Autodesk Inventor part; units mm, degrees
ref_plane "YZ Plane" through (0, 0, 0) normal (1, 0, 0) x (0, 1, 0)
ref_plane "XZ Plane" through (0, 0, 0) normal (0, 1, 0) x (-1, 0, 0)
ref_plane "XY Plane" through (0, 0, 0) normal (0, 0, 1) x (1, 0, 0)
sketch "Sketch1" plane through (0, 0, 0) normal (0, 0, 1) x (1, 0, 0)
  line L0 (-11, -29.75) -> (11, -29.75) construction
  line L1 (14.5, -26.25) -> (14.5, 26.25) construction
  line L2 (11, 29.75) -> (-11, 29.75) construction
  line L3 (-14.5, 26.25) -> (-14.5, -26.25) construction
  line L4 (-14.5, -29.75) -> (14.5, 29.75) construction
  line L5 (14.5, -29.75) -> (-14.5, 29.75) construction
  arc A0 (-11, 29.75) -> (-14.5, 26.25) centre (-11, 26.25) ccw construction
  arc A1 (14.5, 26.25) -> (11, 29.75) centre (11, 26.25) ccw construction
  arc A2 (11, -29.75) -> (14.5, -26.25) centre (11, -26.25) ccw
  arc A3 (-14.5, -26.25) -> (-11, -29.75) centre (-11, -26.25) ccw construction
  line L6 (-17.6, -35) -> (17.6, -35)
  line L7 (20.1, -32.5) -> (20.1, 34.5)
  line L8 (17.6, 37) -> (-17.6, 37)
  line L9 (-20.1, 34.5) -> (-20.1, -32.5)
  line L10 (-20.1, -35) -> (20.1, 37) construction
  line L11 (20.1, -35) -> (-20.1, 37) construction
  line L12 (-20.1, 34.5) -> (-17.6, 37)
  line L13 (-20.1, -32.5) -> (-17.6, -35)
  line L14 (17.6, -35) -> (20.1, -32.5)
  line L15 (17.6, 37) -> (20.1, 34.5)
  circle A4 centre (0, -15.25) radius 14 construction
  circle A5 centre (-17.3, -19.25) radius 1.3
  circle A6 centre (-17.3, 2.75) radius 1.3
  circle A7 centre (-17.3, 24.75) radius 1.3
  circle A8 centre (-11, 32.55) radius 1.3
  line L16 (0, -15.25) -> (0, -1.25) construction
  circle A9 centre (17.3, -19.25) radius 1.3
  circle A10 centre (17.3, 2.75) radius 1.3
  circle A11 centre (17.3, 24.75) radius 1.3
  circle A12 centre (11, 32.55) radius 1.3
  line L17 (-11, 30) -> (11, 30)
  arc A13 (14.75, 26.25) -> (11, 30) centre (11, 26.25) ccw
  line L18 (14.75, 26.25) -> (14.75, -26.25)
  arc A14 (11, -30) -> (14.75, -26.25) centre (11, -26.25) ccw
  line L19 (11, -30) -> (-11, -30)
  arc A15 (-14.75, -26.25) -> (-11, -30) centre (-11, -26.25) ccw
  line L20 (-14.75, -26.25) -> (-14.75, 26.25)
  arc A16 (-11, 30) -> (-14.75, 26.25) centre (-11, 26.25) ccw
  point P0 (0, 0)
  point P1 (0, 1)
  point P2 (0, 29.75)
  dimension "d14" = 28
  dimension "d0" = 29
  dimension "d1" = 59.5
  dimension "d2" = 3.5
  dimension "d3" = 40.2
  dimension "d4" = 72
  dimension "d6" = 2.5
  dimension "d7" = 2.5
  dimension "d8" = 2.5
  dimension "d9" = 2.5
  dimension "d10" = 2.5
  dimension "d11" = 2.5
  dimension "d12" = 2.5
  dimension "d13" = 2.5
  dimension "d15" = 45
  dimension "d16" = 2.6
  dimension "d17" = 17.3
  dimension "d18" = 4
  dimension "d19" = 2.6
  dimension "d20" = 22
  dimension "d21" = 2.6
  dimension "d22" = 22
  dimension "d24" = 2.6
  dimension "d26" = 7.8
  dimension "d27" = 11
  dimension "d28" = 1
  dimension "d51" = 0.25
extrude "Extrusion1" add sketch "Sketch1" along normal blind 6
sketch "Sketch2" plane through (0, 0, 6) normal (0, 0, 1) x (1, 0, 0)
  line L0 (26.1, 28) -> (26.1, 20)
  line L1 (20.1, -32.5) -> (20.1, 34.5)
  line L2 (26.1, 20) -> (20.1, 20)
  line L3 (26.1, 28) -> (20.1, 28)
  line L4 (-14.5, 0) -> (14.5, 0) construction
  line L5 (0, 29.4068) -> (0, -29.4068) construction
  line L6 (-26.1, 28) -> (-26.1, 20)
  line L7 (-26.1, 20) -> (-20.1, 20)
  line L8 (-26.1, 28) -> (-20.1, 28)
  line L9 (26.1, -28) -> (26.1, -20)
  line L10 (26.1, -20) -> (20.1, -20)
  line L11 (26.1, -28) -> (20.1, -28)
  line L12 (-26.1, -20) -> (-20.1, -20)
  line L13 (-26.1, -28) -> (-26.1, -20)
  line L14 (-26.1, -28) -> (-20.1, -28)
  line L15 (-20.1, 28) -> (-20.1, 20)
  line L16 (-20.1, 34.5) -> (-20.1, -32.5)
  line L17 (-20.1, -20) -> (-20.1, -28)
  line L18 (-20.1, 34.5) -> (-20.1, -32.5)
  point P0 (0, 0)
  point P1 (26.1, 24)
  point P2 (20.1, -20)
  point P3 (20.1, -28)
  point P4 (0, 0)
  dimension "d31" = 24
  dimension "d32" = 8
  dimension "d33" = 6
extrude "Extrusion2" add sketch "Sketch2" against normal up to surface (6 mm away)
fillet "Fillet1" radius 5 8 edges at (20.1, 28, 3) (-20.1, 28, 3) (-20.1, -20, 3) (-20.1, -28, 3) (20.1, -28, 3) (20.1, 20, 3) (20.1, -20, 3) (-20.1, 20, 3)
sketch "Sketch3" plane through (-26.1, 20, 6) normal (-1, 0, 0) x (0, 0, 1)
  line L0 (-6, 0) -> (-6, 8) construction
  line L1 (0, 0) -> (-6, 0) construction
  line L2 (0, 8) -> (0, 0) construction
  line L3 (0, 8) -> (-6, 8) construction
  line L4 (0, 8) -> (-6, 0) construction
  circle A0 centre (-3, 4) radius 2
  line L5 (-6, -48) -> (-6, -40) construction
  line L6 (0, -48) -> (-6, -48) construction
  line L7 (0, -40) -> (0, -48) construction
  line L8 (0, -40) -> (-6, -40) construction
  line L9 (0, -40) -> (-6, -48) construction
  circle A1 centre (-3, -44) radius 2
  point P0 (-6, -20)
  dimension "d37" = 4
  dimension "d38" = 4
extrude "Extrusion3" cut sketch "Sketch3" against normal blind 6
mirror "Mirror1" about plane through (0, 0, 0) normal (1, 0, 0) of "Extrusion3"
thread "Thread1"
thread "Thread2"
thread "Thread3"
thread "Thread4"
equation "\"d7\" = d6"
equation "\"d8\" = d6"
equation "\"d9\" = d8"
equation "\"d10\" = d6"
equation "\"d11\" = d10"
equation "\"d12\" = d6"
equation "\"d13\" = d12"
properties part number "DynamixelServoMount" material "Aluminum 6061"
Can you work these out from the model? Positions are in its coordinate system, mm. A direction names the side the tool comes from. Coordinates: 2 decimals unless noted, no trailing zeros. Write each loop counter-clockwise with the first axis right and the second up, starting at its lowest first coordinate (ties: lowest second). Pieces come first, ordered by that corner, then holes.
Q1. Which directions (+Z, -Z, +X, -X, +Y, -Y) give clear straight access to the entire face, cutting with the end or side of a thin tool? Please do faces 1 (the face through (14.75, 0, 3)), 2 (the face through (20.1, 24, 3)), 3 (the face through (0, -35, 3)), 4 (the face through (-21.53, 18.5, 3.04)), 5 (the face through (-20.1, 34, 3)).
Results found:
face 1: +Z, -Z
face 2: +X
face 3: +Z, -Z, +X, -X, -Y
face 4: +Z, -Z, -X
face 5: +Z, -Z, -X, +Y
Q2. Imagine slicing it at B-B, the plane x = 21. List the corners of the cut face in (y, z) for me.
Results found:
outline: (-30.1, 0) - (-17.86, 0) - (-17.86, 6) - (-30.1, 6) - close; (17.86, 0) - (30.14, 0) - (30.14, 6) - (17.86, 6) - close; hole circle Ø4 at (-24, 3); hole circle Ø4 at (24, 3)
Q3. If we mould it in two halves opening along X, with no side actions, what happens to faces 6 (the face through (-16.7, -18.097, 2.958)), 7 (the face through (-26.1, 23, 5)), 8 (the face through (-16, 1, 0))? For each: +X half, -X half, draft (parallel to the pull), parting line (faces both ways), or undercut.
Results found:
face 6: undercut
face 7: -X half
face 8: draft
Q4. Imagine slicing it at C-C, the plane x = 8. List the corners of the cut face in (y, z) for me.
Results found:
outline: (-35, 0) - (-30, 0) - (-30, 6) - (-35, 6) - close; (30, 0) - (37, 0) - (37, 6) - (30, 6) - close
Q5. Please list where these lines run through material, in increasing order: L1, parallel to Y at x = 17.3, z = 1.95; L2, parallel to Y at x = 3, z = 3.4; L3, parallel to X at y = -21, z = 4.15.
Results found:
L1: y = -35 to -20.55, -17.95 to 1.45, 4.05 to 23.45, 26.05 to 37
L2: y = -35 to -30, 30 to 37
L3: x = -26.1 to -14.75, 14.75 to 26.1
Q6. For P1, Ø2, axis at y = 24, z = 3.5, coming from the -X side; P2, Ø0.8, axis at x = 25.5, z = 3, coming from the +Y side; P3, Ø1.5, axis at y = 12, z = 5, coming from the +X side, each with a flat end and sliding along its axis, tell me the tip position at first contact or that it passes through.
Results found:
P1: stops at x = -20.1
P2: stops at y = 28
P3: stops at x = 20.1
Q7. Imagine slicing it at A-A, the plane y = -24. List the corners of the cut face in (x, z) for me, plus the area to 3 significant figures.
Results found:
outline: (-26.1, 0) - (-14.75, 0) - (-14.75, 6) - (-26.1, 6) - (-26.1, 5) - (-20.1, 5) - (-20.1, 1) - (-26.1, 1) - close; (14.75, 0) - (26.1, 0) - (26.1, 1) - (20.1, 1) - (20.1, 5) - (26.1, 5) - (26.1, 6) - (14.75, 6) - close
area: 88.2 mm2
Q8. Imagine slicing it at D-D, the plane y = 24.75. List the corners of the cut face in (x, z) for me.
Results found:
outline: (-26.1, 0) - (-18.6, 0) - (-18.6, 6) - (-26.1, 6) - (-26.1, 4.85) - (-20.1, 4.85) - (-20.1, 1.15) - (-26.1, 1.15) - close; (-16, 0) - (-14.75, 0) - (-14.75, 6) - (-16, 6) - close; (14.75, 0) - (16, 0) - (16, 6) - (14.75, 6) - close; (18.6, 0) - (26.1, 0) - (26.1, 1.15) - (20.1, 1.15) - (20.1, 4.85) - (26.1, 4.85) - (26.1, 6) - (18.6, 6) - close
